Check sheet for the drawn part. Datum: minimum x, y, z corner. Units: mm. Coordinates: 2 decimals unless noted, no trailing zeros. Write each loop counter-clockwise with the first axis right and the second up, starting at its lowest first coordinate (ties: lowest second). Pieces come first, ordered by that corner, then holes. Notation, with made-up numbers: (78, 57) -> (116, 57) arc R19 ccw to (116, 76) -> close; hole circle Ø2 at (41, 36). An arc over 180 degrees is marked (long way). One line per question, with ' | ' between items.
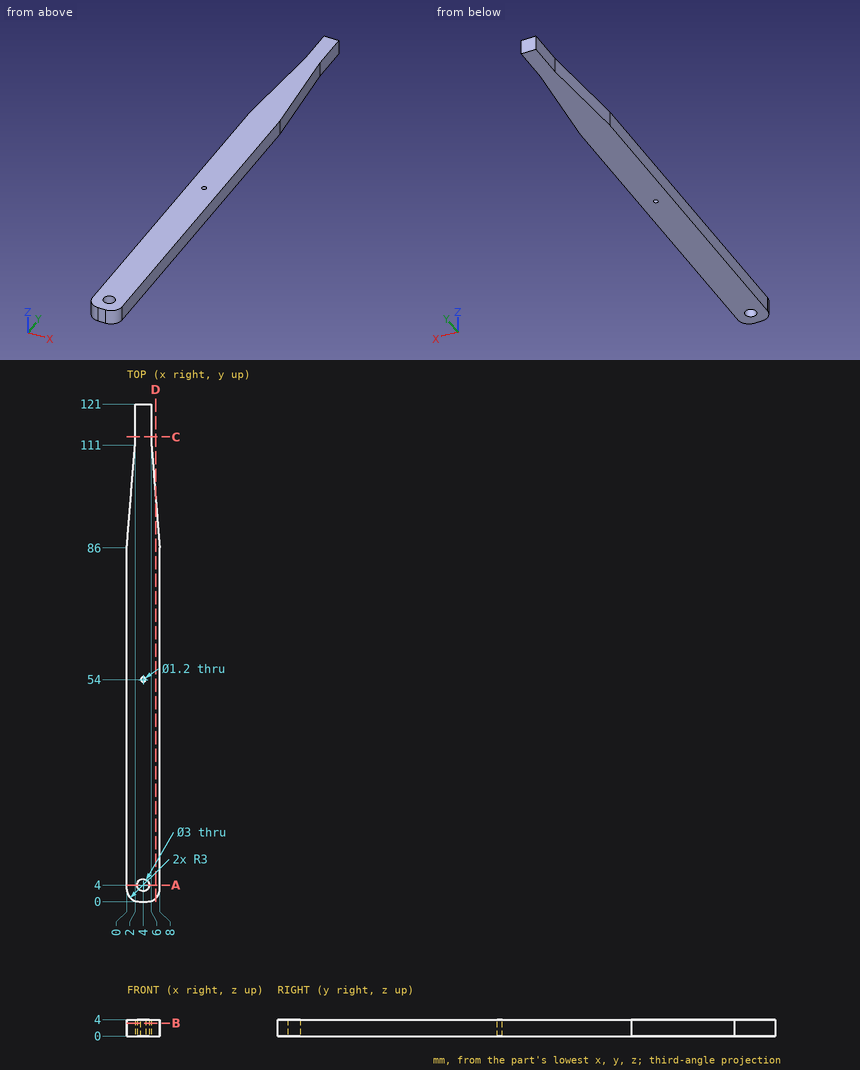
1. Cross-section at C-C on y = 113. Record the boundary of the cut face in (x, z).
Worked answers:
outline: (2, 0) -> (6, 0) -> (6, 4) -> (2, 4) -> close
2. Cross-section at A-A on y = 4. Record the boundary of the cut face in (x, z), and give its area (3 significant figures).
Worked answers:
outline: (0, 0) -> (2.5, 0) -> (2.5, 4) -> (0, 4) -> close; (5.5, 0) -> (8, 0) -> (8, 4) -> (5.5, 4) -> close | area: 20.0 mm²
3. Cross-section at D-D on x = 7. Record the boundary of the cut face in (y, z).
Worked answers:
outline: (0.76, 0) -> (98.5, 0) -> (98.5, 4) -> (0.76, 4) -> close
4. Go/stop test with flat-tipped pins: P1, Ø2, axis at x = 4, z = 2, coming from the -Y side; P2, Ø0.7, axis at x = 4, y = 54, coming from the -Z side. Record where each tip stops, or that it passes through.
Worked answers:
P1: y = 0 | P2: through
5. Cross-section at B-B on z = 3.1. Record the boundary of the cut face in (x, y).
Worked answers:
outline: (0, 3) arc R3 ccw to (3, 0) -> (5, 0) arc R3 ccw to (8, 3) -> (8, 86) -> (6, 111) -> (6, 121) -> (2, 121) -> (2, 111) -> (0, 86) -> close; hole circle Ø3 at (4, 4); hole circle Ø1.2 at (4, 54)
6. Material ranges on line 1 (Y direction, x = 4, z = 1.7); line 2 (Y direction, x = 4.5, z = 3.45); line 3 (X direction, y = 54, z = 2.45), recorded low to high. Write a range as from..to.
Worked answers:
line 1: 0..2.5, 5.5..53.4, 54.6..121 | line 2: 0..2.59, 5.41..53.67, 54.33..121 | line 3: 0..3.4, 4.6..8
